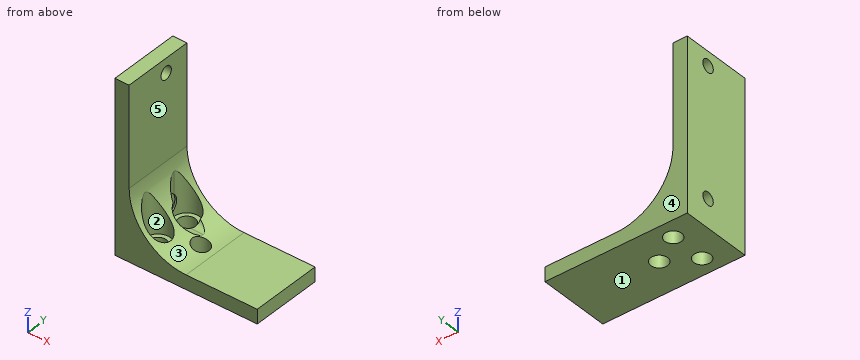
from build123d import *

# Parameters (mm, degrees)
CROQUIS1_W                   = 50
CROQUIS1_H                   = 25
CROQUIS1_R                   = 2.95
SALIENTE_EXTRUIR1_DEPTH      = 5
CROQUIS1_3_W                 = 5
CROQUIS1_3_H                 = 25
SALIENTE_EXTRUIR2_DEPTH      = 60
REDONDEO2_DEPTH              = 25
REDONDEO2_START              = 5
REDONDEO2_2_OUTLINE_R        = 2.95
REDONDEO2_2_DEPTH            = 20
CROQUIS4_R                   = 4.45
CORTAR_EXTRUIR1_DEPTH        = 79.421935739
CROQUIS5_R                   = 2.25
CORTAR_EXTRUIR2_DEPTH        = 80.056941536
CROQUIS5_3_R                 = 3.75
CROQUIS5_3_R_2               = 2.25
CORTAR_EXTRUIR_L_MINA3_DEPTH = 80.056941536


with BuildPart() as part:
    # Croquis1 → Saliente-Extruir1 (new body)
    with BuildSketch(Plane.XY):
        with Locations((25, 12.5)):
            Rectangle(CROQUIS1_W, CROQUIS1_H)
        with Locations((10, 18.75)):
            Circle(CROQUIS1_R, mode=Mode.SUBTRACT)
        with Locations((10, 6.25)):
            Circle(CROQUIS1_R, mode=Mode.SUBTRACT)
        with Locations((20, 12.5)):
            Circle(CROQUIS1_R, mode=Mode.SUBTRACT)
    extrude(amount=SALIENTE_EXTRUIR1_DEPTH)

    # Croquis1<3> → Saliente-Extruir2 (add)
    with BuildSketch(Plane.XY):
        with Locations((2.5, 12.5)):
            Rectangle(CROQUIS1_3_W, CROQUIS1_3_H)
    extrude(amount=SALIENTE_EXTRUIR2_DEPTH)

    # Redondeo2: read off the stored shape, not the designer's step
    # Redondeo2 outline → Redondeo2 (add)
    with BuildSketch(Plane(origin=(0, 0, 0), x_dir=(1, 0, 0), z_dir=(0, 1, 0))):
        with BuildLine():
            Line((5, -5), (5, -25))
            ThreePointArc((5, -25), (10.857864376, -10.857864376), (25, -5))
            Line((25, -5), (5, -5))
        make_face()
    extrude(amount=REDONDEO2_DEPTH)

    # Redondeo2 2 outline → Redondeo2 2 (cut)
    with BuildSketch(Plane.XY.offset(REDONDEO2_START)):
        with Locations((10, 18.75)):
            Circle(REDONDEO2_2_OUTLINE_R)
        with Locations((20, 12.5)):
            Circle(REDONDEO2_2_OUTLINE_R)
        with Locations((10, 6.25)):
            Circle(REDONDEO2_2_OUTLINE_R)
    extrude(amount=REDONDEO2_2_DEPTH, mode=Mode.SUBTRACT)

    # Croquis4 → Cortar-Extruir1 (cut, through all)
    with BuildSketch(Plane.XY.offset(5)):
        with Locations(Location((10, 18.75, 0), (0, 0, 180))):
            Circle(CROQUIS4_R)
        with Locations(Location((10, 6.25, 0), (0, 0, 180))):
            Circle(CROQUIS4_R)
    extrude(amount=CORTAR_EXTRUIR1_DEPTH, mode=Mode.SUBTRACT)

    # Croquis5 → Cortar-Extruir2 (cut, through all)
    with BuildSketch(Plane(origin=(5, 0, 0), x_dir=(0, 0, -1), z_dir=(1, 0, 0))):
        with Locations(Location((-55, 16, 0), (0, 0, 90))):
            Circle(CROQUIS5_R)
        with Locations(Location((-10, 16, 0), (0, 0, 90))):
            Circle(CROQUIS5_R)
    extrude(amount=-CORTAR_EXTRUIR2_DEPTH, mode=Mode.SUBTRACT)

    # Croquis5<3> → Cortar-Extruir-Lámina3 (cut, through all)
    with BuildSketch(Plane(origin=(5, 0, 0), x_dir=(0, 0, -1), z_dir=(1, 0, 0))):
        with Locations((-10, 16)):
            Circle(CROQUIS5_3_R)
        with Locations((-10, 16)):
            Circle(CROQUIS5_3_R_2, mode=Mode.SUBTRACT)
    extrude(amount=CORTAR_EXTRUIR_L_MINA3_DEPTH, mode=Mode.SUBTRACT)


with BuildPart() as cortar_extruir_l_mina3_kept_piece:
    # of the separate pieces the step leaves, the one the design keeps (cortar_extruir_l_mina3_pieces_kept)
    add(part.part.solids().sort_by_distance((0, 0, 0))[0])


solid = cortar_extruir_l_mina3_kept_piece.part
Model file for the job. Use its own axes, mm. Face numbers are marked on the shaded views. A direction names the side the tool comes from. Give positions to 0.01 mm unless a question says otherwise; leave off trailing zeros. Loops run counter-clockwise (first coordinate to the right, second up) from the corner with the lowest first, then second, coordinate; pieces in that order, holes last.
Item 1: Slice it at D-D (y = 6.25). Write the cut outline in (x, z), plus the area to 3 significant figures.
Check values:
outline: (0, 0) - (7.05, 0) - (7.05, 5) - (5.55, 5) - (5.55, 20.34) arc R20 cw to (5, 25) - (5, 60) - (0, 60) - close; (12.95, 0) - (50, 0) - (50, 5) - (25, 5) arc R20 cw to (14.45, 8.01) - (14.45, 5) - (12.95, 5) - close
area: 515 mm2
Item 2: Slice it at B-B (x = 10). Write the cut outline in (y, z).
Check values:
outline: (0, 0) - (3.3, 0) - (3.3, 5) - (1.8, 5) - (1.8, 11.77) - (0, 11.77) - close; (9.2, 0) - (15.8, 0) - (15.8, 5) - (14.3, 5) - (14.3, 6.66) arc R3.75 cw to (12.69, 11.77) - (10.7, 11.77) - (10.7, 5) - (9.2, 5) - close; (21.7, 0) - (25, 0) - (25, 11.77) - (23.2, 11.77) - (23.2, 5) - (21.7, 5) - close
Item 3: Mould opens along X. For the marked faces 1, 2 and 3 say: +X half, -X half, draft (parallel to the pull), parting line (faces both ways), or undercut.
Check values:
face 1: draft
face 2: undercut
face 3: +X half
Item 4: Which spindle directions (+Z, -Z, +X, -X, +Y, -Y) get a long thin tool onto all of the face, cutting with end or side? Do the marked faces 4 and 5. Say none if no direction does.
Check values:
face 4: +Z, -Z, +X, -X, +Y
face 5: +Z, +X, +Y, -Y
Item 5: Slice it at A-A (z = 55). Write the cut outline in (x, y).
Check values:
outline: (0, 0) - (5, 0) - (5, 13.75) - (0, 13.75) - close; (0, 18.25) - (5, 18.25) - (5, 25) - (0, 25) - close
Item 6: Slice it at C-C (x = 20). Write the cut outline in (y, z).
Check values:
outline: (0, 0) - (9.55, 0) - (9.55, 5.64) - (0, 5.64) - close; (15.45, 0) - (25, 0) - (25, 5.64) - (15.45, 5.64) - close
Item 7: Drill centre lines: line 1 along Y through (x, z) = (10, 1); line 2 along Z through (x, y) = (1.3, 16); line 3 along Y through (x, z) = (10, 10). Where is each one in solid material? Low to high.
Check values:
line 1: y = 0 to 3.3, 9.2 to 15.8, 21.7 to 25
line 2: z = 0 to 7.75, 12.25 to 52.75, 57.25 to 60
line 3: y = 0 to 1.8, 10.7 to 12.25, 23.2 to 25
Item 8: Drop flat-ended pins along their axis: P1, Ø7, axis at x = 20, y = 12.5, coming from the -Z side; P2, Ø6, axis at y = 15.5, z = 10, coming from the +X side; P3, Ø8, axis at x = 11.5, y = 16, coming from the +Z side; P4, Ø2, axis at x = 42, y = 19, coming from the +Z side. Give the stop position or say it passes through.
Check values:
P1: stops at z = 0
P2: stops at x = 5
P3: stops at z = 15.08
P4: stops at z = 5
